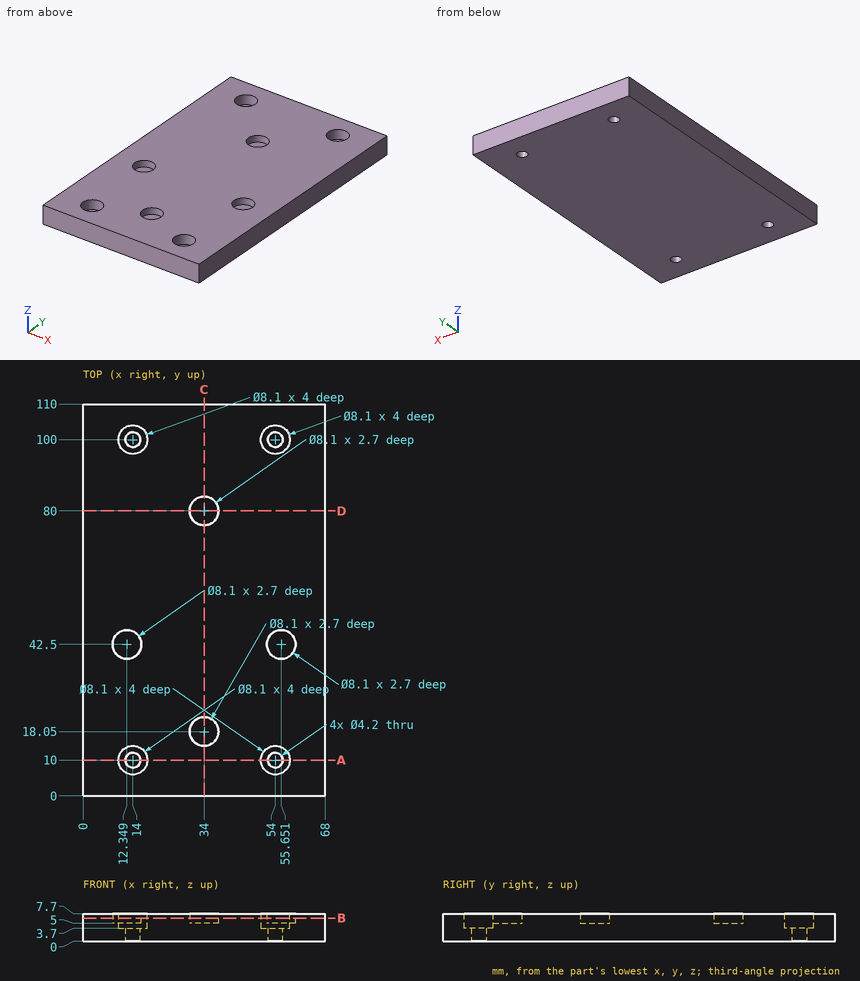
Geometry: see drawing. Coordinates: mm, zero at the bounding-box minimum. Round coordinates to 2 decimals unless told otherwise and drop trailing zeros. Order: outer loops, then holes, each group sorted by start corner. A loop starts at its lowest first (then second) coordinate and runs counter-clockwise, first axis right, second up. Notation, with made-up numbers: (63, 21) - (112, 21) arc R24 cw to (112, 55) - close; hole circle Ø4 at (11, 32). An arc over 180 degrees is marked (long way). One line per question, with ' | ' between items. Start each with the question number.
1) Cut plane B-B, the plane z = 6.5. Give the number of separate pieces and of enclosed holes in the cut face, then the cut area to 3 significant figures.
2) Cut plane C-C, the plane x = 34. Return the cut outline in (y, z), then the cut area to 3 significant figures.
3) Cut plane A-A, the plane y = 10. Return the cut outline in (x, z), then the cut area to 3 significant figures.
4) Contact query for a flat-ended pin moving along its axis: P1, Ø6.5, axis at x = 54, y = 100, coming from the +Z side. Output: stop coordinate, or through.
5) Ray query, probe 1 along X at (y, z) = (10, 2.45); probe 2 along X at (y, z) = (42.5, 6.85); probe 3 along X at (y, z) = (18.05, 6.6). Return the intervals inside material, ascending.
6) Cut plane D-D, the plane y = 80. Return the cut outline in (x, z).
Worked out:
1) separate pieces: 1 | enclosed holes: 8 | area: 7,070 mm^2
2) outline: (0, 0) - (110, 0) - (110, 7.7) - (84.05, 7.7) - (84.05, 5) - (75.95, 5) - (75.95, 7.7) - (22.1, 7.7) - (22.1, 5) - (14, 5) - (14, 7.7) - (0, 7.7) - close | area: 803 mm^2
3) outline: (0, 0) - (11.9, 0) - (11.9, 3.7) - (9.95, 3.7) - (9.95, 7.7) - (0, 7.7) - close; (16.1, 0) - (51.9, 0) - (51.9, 3.7) - (49.95, 3.7) - (49.95, 7.7) - (18.05, 7.7) - (18.05, 3.7) - (16.1, 3.7) - close; (56.1, 0) - (68, 0) - (68, 7.7) - (58.05, 7.7) - (58.05, 3.7) - (56.1, 3.7) - close | area: 428 mm^2
4) P1: stops at z = 3.7
5) probe 1: x = 0 to 11.9, 16.1 to 51.9, 56.1 to 68 | probe 2: x = 0 to 8.3, 16.4 to 51.6, 59.7 to 68 | probe 3: x = 0 to 29.95, 38.05 to 68
6) outline: (0, 0) - (68, 0) - (68, 7.7) - (38.05, 7.7) - (38.05, 5) - (29.95, 5) - (29.95, 7.7) - (0, 7.7) - close
